```python
from build123d import *

# Parameters (mm, degrees)
SKETCH1_W           = 50.8
SKETCH1_H           = 50.8
SKETCH1_W_2         = 44.45
SKETCH1_H_2         = 44.45
BOSS_EXTRUDE1_DEPTH = 965.2
SKETCH2_R           = 3.302
CUT_EXTRUDE1_DEPTH  = 51.8


with BuildPart() as part:
    # Sketch1 → Boss-Extrude1 (new body)
    with BuildSketch(Plane.XY):
        with Locations((0, 25.4)):
            Rectangle(SKETCH1_W, SKETCH1_H)
        with Locations((0, 25.4)):
            Rectangle(SKETCH1_W_2, SKETCH1_H_2, mode=Mode.SUBTRACT)
    extrude(amount=BOSS_EXTRUDE1_DEPTH)

    # Sketch2 → Cut-Extrude1 (cut, through all)
    with BuildSketch(Plane(origin=(0, 50.8, 0), x_dir=(1, 0, 0), z_dir=(0, 1, 0))):
        with Locations((0, -215.9)):
            Circle(SKETCH2_R)
        with Locations((0, -479.425)):
            Circle(SKETCH2_R)
        with Locations((0, -742.95)):
            Circle(SKETCH2_R)
    extrude(amount=-CUT_EXTRUDE1_DEPTH, mode=Mode.SUBTRACT)


solid = part.part
```
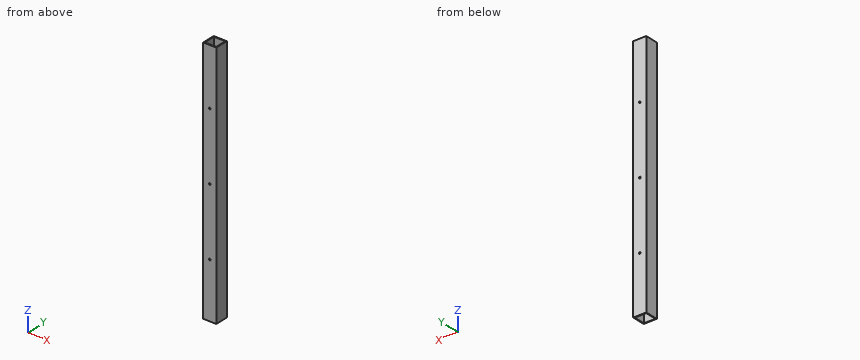
Work out the finished part from the listing and answer in its coordinate system (mm). Coordinates: 2 decimals unless noted, no trailing zeros. Write each loop counter-clockwise with the first axis right and the second up, starting at its lowest first coordinate (ties: lowest second). Pieces come first, ordered by that corner, then holes.
Q1. This flat-tipped pin is pushed along its axis until it touches: pin 1 Ø7.5 at (x, z) = (0, 215.9) entering from -Y. Where does it stop, or does it pass through?
Q2. A cutting plane is placed at B-B, the plane z = 113. Give the vertices of the cut face in (x, y) (3 decimals).
Q3. A cutting plane is placed at A-A, the plane y = 22. Give the vertices of the cut face in (x, z) (3 decimals).
Q4. Find the intervals of material crossed by line 1 (Z direction, x = 0, y = 1.1); line 2 (X direction, y = 26.5, z = 142) (3 decimals); line 3 (Y direction, x = 5, z = 677) (3 decimals), in increasing order.
Findings below:
1. pin 1: stops at y = 0
2. outline: (-25.4, 0) - (25.4, 0) - (25.4, 50.8) - (-25.4, 50.8) - close; hole (-22.225, 3.175) - (22.225, 3.175) - (22.225, 47.625) - (-22.225, 47.625) - close
3. outline: (-25.4, 0) - (-22.225, 0) - (-22.225, 965.2) - (-25.4, 965.2) - close; (22.225, 0) - (25.4, 0) - (25.4, 965.2) - (22.225, 965.2) - close
4. line 1: z = 0 to 212.6, 219.2 to 476.12, 482.73 to 739.65, 746.25 to 965.2
4. line 2: x = -25.4 to -22.225, 22.225 to 25.4
4. line 3: y = 0 to 3.175, 47.625 to 50.8
